Autodesk Inventor part; units mm, degrees
ref_plane "YZ Plane" through (0, 0, 0) normal (1, 0, 0) x (0, 1, 0)
ref_plane "XZ Plane" through (0, 0, 0) normal (0, 1, 0) x (-1, 0, 0)
ref_plane "XY Plane" through (0, 0, 0) normal (0, 0, 1) x (1, 0, 0)
sketch "Sketch1" plane through (0, 0, 0) normal (0, 1, 0) x (-1, 0, 0)
  circle A0 centre (0, 0) radius 2
  circle A1 centre (0, 0) radius 3
  dimension "d0" = 4
  dimension "d1" = 6
extrude "Extrusion1" add sketch "Sketch1" along normal blind 20
sketch "Sketch2" plane through (0, 20, 0) normal (0, 1, 0) x (1, 0, 0)
  circle A0 centre (0, 0) radius 3
  circle A1 centre (0, 0) radius 2
  line L0 (10, -5) -> (10, 5)
  dimension "d4" = 10
  dimension "d5" = 5
  dimension "d6" = 10
revolve "Revolution1" add sketch "Sketch2" angle 90 about axis through (10, 20, 5) along (0, 0, -1)
sketch "Sketch3" plane through (10, 30, 0) normal (1, 0, 0) x (0, 0, -1)
  circle A0 centre (0, 0) radius 3
  circle A1 centre (0, 0) radius 2
  point P0 (0, -30)
extrude "Extrusion2" add sketch "Sketch3" along normal blind 200
properties part number "Pipe"
Source: CAD feature listing. Evaluate the final solid. Frame: model axes, mm. A direction names the side the tool comes from. Round coordinates to 2 decimals unless told otherwise and drop trailing zeros. Write each loop counter-clockwise with the first axis right and the second up, starting at its lowest first coordinate (ties: lowest second). Pieces come first, ordered by that corner, then holes. Notation, with made-up numbers: M 78,-6 L 133,-6 A25 ccw 133,18 Z; hole C 40.25,-5.5 d8. An arc over 180 degrees is marked long. Answer as a JSON object with one key per item and string values. Group by question number.
(1) First-contact query: pin 1 (3 mm diameter, centred on y = 21, z = 2, fed in from -X); pin 2 (1.5 mm diameter, centred on x = 75, z = -2, fed in from -Y); pin 3 (2 mm diameter, centred on x = 63.5, z = 1.5, fed in from +Y). Flat tips, straight axial feed; report the tip coordinate or a pass-through.
(2) Section query B-B on x = 27. Output: boundary loops of the cut face in (y, z).
(3) Section query A-A on z = 0. Output: boundary loops of the cut face in (x, y).
(4) Reachability of faces 5 (the flat face through (-1, 0, -2)), 6 (the cylindrical face through (108.6, 32.93, 0.65)) from +Z, -Z, +X, -X, +Y, -Y: full face, straight path, thin tool, end or side. Return the list, or none.
(5) Ray query, line 1 (Z direction, x = 0, y = 15.5); line 2 (Y direction, x = 98, z = 0.25). Return the intervals inside material, ascending. Write a range as [from, to].
(6) Mould query, pull axis X, two halves, no side actions, for faces 1 (the cylindrical face through (109, 32, 0)), 2 (the cylindrical face through (0, 10, 2)), 3 (the cylindrical face through (3, 10, 0)), 4 (the flat face through (210, 28, -1)). Classes: +X half, -X half, draft (parallel to the pull), parting line (faces both ways), or undercut.
(7) Section query C-C on y = 5.5. Output: boundary loops of the cut face in (x, z).
Computed values:
{
 "1": {"pin 1": "x = -2.93", "pin 2": "y = 27.27", "pin 3": "y = 32.96"},
 "2": {"outline": "C 30,0 d6; hole C 30,0 d4"},
 "3": {"outline": "M -3,0 L -2,0 L -2,20 A12 cw 10,32 L 210,32 L 210,33 L 10,33 A13 ccw -3,20 Z; M 2,0 L 3,0 L 3,20 A7 cw 10,27 L 210,27 L 210,28 L 10,28 A8 ccw 2,20 Z"},
 "4": {"face 5": "+Z, -Z, +X, -X, -Y", "face 6": "+X"},
 "5": {"line 1": "[-3, -2], [2, 3]", "line 2": "[27.01, 28.02], [31.98, 32.99]"},
 "6": {"face 1": "draft", "face 2": "undercut", "face 3": "parting line", "face 4": "+X half"},
 "7": {"outline": "C 0,0 d6; hole C 0,0 d4"}
}
